Geometry check sheet. Reference: drawing and pictorial views, mm from the part's lowest x, y, z. Coordinates: 2 decimals unless noted, no trailing zeros. Write each loop counter-clockwise with the first axis right and the second up, starting at its lowest first coordinate (ties: lowest second). Pieces come first, ordered by that corner, then holes. Notation, with made-up numbers: (28.25, 9.25) -> (76.25, 9.25) arc R27 ccw to (76.25, 42.25) -> close; hole circle Ø6 at (-23.75, -32.5). An arc over 180 degrees is marked (long way). Use a Markdown table: item, result.
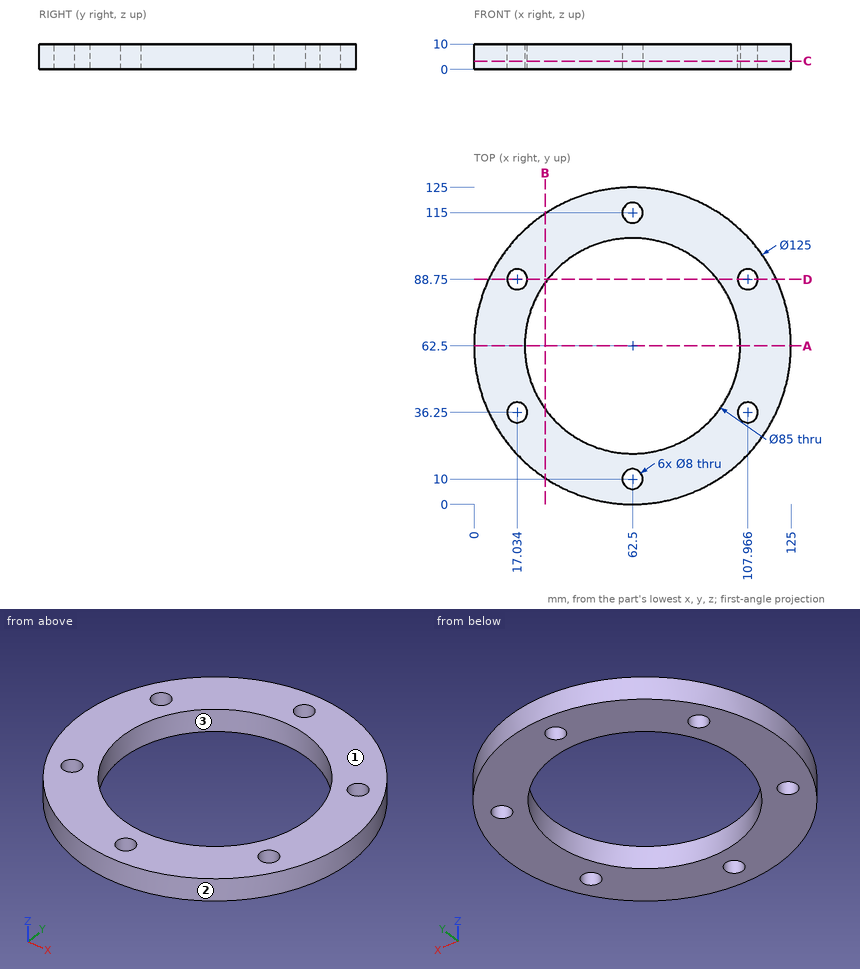
Item 1: Section check C-C on z = 3.25. Record the boundary of the cut face in (x, y).
Answer block:
| item | result |
|---|---|
| outline | circle Ø125 at (62.5, 62.5); hole circle Ø8 at (17.03, 36.25); hole circle Ø8 at (17.03, 88.75); hole circle Ø85 at (62.5, 62.5); hole circle Ø8 at (62.5, 10); hole circle Ø8 at (62.5, 115); hole circle Ø8 at (107.97, 36.25); hole circle Ø8 at (107.97, 88.75) |
Item 2: Depth check by flat-ended pin: P1, Ø1, axis at x = 23, z = 8, coming from the +Y side; P2, Ø5, axis at x = 17.03, y = 88.75, coming from the +Z side; P3, Ø4, axis at x = 107.5, z = 2, coming from the -Y side; P4, Ø1.5, axis at y = 108, z = 8.5, coming from the +X side. Enter the tip coordinate at first touch or a pass-through.
Answer block:
| item | result |
|---|---|
| P1 | stops at y = 111.34 |
| P2 | passes through |
| P3 | stops at y = 17.14 |
| P4 | stops at x = 106.13 |
Item 3: Section check A-A on y = 62.5. Record the boundary of the cut face in (x, z), then the cut area to 3 significant figures.
Answer block:
| item | result |
|---|---|
| outline | (0, 0) -> (20, 0) -> (20, 10) -> (0, 10) -> close; (105, 0) -> (125, 0) -> (125, 10) -> (105, 10) -> close |
| area | 400 mm^2 |
Item 4: Section check B-B on x = 28. Record the boundary of the cut face in (y, z) (1 decimal).
Answer block:
| item | result |
|---|---|
| outline | (10.4, 0) -> (37.7, 0) -> (37.7, 10) -> (10.4, 10) -> close; (87.3, 0) -> (114.6, 0) -> (114.6, 10) -> (87.3, 10) -> close |
Item 5: Mould release check, pull along X, two halves, no side actions. Record for the marked faces 1, 2 and 3: +X half, -X half, draft (parallel to the pull), parting line (faces both ways), or undercut.
Answer block:
| item | result |
|---|---|
| face 1 | draft |
| face 2 | parting line |
| face 3 | undercut |
Item 6: Thickness scan on L1, parallel to Y at x = 62.5, z = 5.5; L2, parallel to X at y = 86, z = 7.5 (1 decimal); L3, parallel to Y at x = 59, z = 7.75 (1 decimal). Record the ranges inside material, lowest first. Write a range as [from, to].
Answer block:
| item | result |
|---|---|
| L1 | y = [0, 6], [14, 20], [105, 111], [119, 125] |
| L2 | x = [4.6, 14.1], [19.9, 27.1], [97.9, 105.1], [110.9, 120.4] |
| L3 | y = [0.1, 8.1], [11.9, 20.1], [104.9, 113.1], [116.9, 124.9] |
Item 7: Section check D-D on y = 88.75. Record the boundary of the cut face in (x, z) (1 decimal), then the cut area to 3 significant figures.
Answer block:
| item | result |
|---|---|
| outline | (5.8, 0) -> (13, 0) -> (13, 10) -> (5.8, 10) -> close; (21, 0) -> (29.1, 0) -> (29.1, 10) -> (21, 10) -> close; (95.9, 0) -> (104, 0) -> (104, 10) -> (95.9, 10) -> close; (112, 0) -> (119.2, 0) -> (119.2, 10) -> (112, 10) -> close |
| area | 306 mm^2 |
